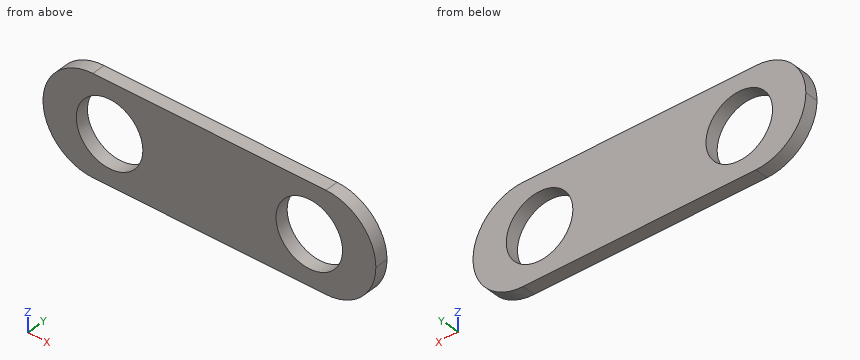
```python
from build123d import *

# Parameters (mm, degrees)
SKETCH1_W           = 50
SKETCH1_H           = 15
BOSS_EXTRUDE1_DEPTH = 2
SKETCH2_R           = 5
CUT_EXTRUDE1_DEPTH  = 2
CUT_EXTRUDE2_DEPTH  = 2


with BuildPart() as part:
    # Sketch1 → Boss-Extrude1 (new body)
    with BuildSketch(Plane(origin=(0, 0, 0), x_dir=(1, 0, 0), z_dir=(0, 1, 0))):
        with Locations((25, 7.5)):
            Rectangle(SKETCH1_W, SKETCH1_H)
    extrude(amount=BOSS_EXTRUDE1_DEPTH)

    # Sketch2 → Cut-Extrude1 (cut)
    with BuildSketch(Plane(origin=(0, 2, 0), x_dir=(1, 0, 0), z_dir=(0, 1, 0))):
        with Locations(Location((10, 7.5, 0), (0, 0, 270))):
            Circle(SKETCH2_R)
        with Locations(Location((40, 7.5, 0), (0, 0, 90))):
            Circle(SKETCH2_R)
    extrude(amount=-CUT_EXTRUDE1_DEPTH, mode=Mode.SUBTRACT)

    # Sketch5 → Cut-Extrude2 (cut)
    with BuildSketch(Plane(origin=(0, 2, 0), x_dir=(1, 0, 0), z_dir=(0, 1, 0))):
        with BuildLine():
            ThreePointArc((0, 7.5), (2.196699141, 12.803300859), (7.5, 15))
            Line((7.5, 15), (0, 15))
            Line((0, 15), (0, 7.5))
        make_face()
        with BuildLine():
            ThreePointArc((7.5, 0), (2.196699141, 2.196699141), (0, 7.5))
            Line((0, 7.5), (0, 0))
            Line((0, 0), (7.5, 0))
        make_face()
        with BuildLine():
            Line((50, 15), (42.5, 15))
            ThreePointArc((42.5, 15), (47.803300859, 12.803300859), (50, 7.5))
            Line((50, 7.5), (50, 15))
        make_face()
        with BuildLine():
            Line((50, 0), (50, 7.5))
            ThreePointArc((50, 7.5), (47.803300859, 2.196699141), (42.5, 0))
            Line((42.5, 0), (50, 0))
        make_face()
    extrude(amount=-CUT_EXTRUDE2_DEPTH, mode=Mode.SUBTRACT)


solid = part.part
```
Geometry: final body of the model. Coordinates: model frame, mm. Give positions to 0.01 mm unless a question says otherwise; leave off trailing zeros. Write each loop counter-clockwise with the first axis right and the second up, starting at its lowest first coordinate (ties: lowest second). Pieces come first, ordered by that corner, then holes.
1. Section query A-A, the plane x = 40. Return loops of the section in (y, z).
2. Section query D-D, the plane z = -9.25. Return loops of the section in (x, y).
3. Line query: probe 1 along X at (y, z) = (0.9, -7.5); probe 2 along X at (y, z) = (1.4, -11.5); probe 3 along Z at (x, y) = (40, 1.4). Output: solid intervals per line, ascending.
4. Section query C-C, the plane z = -5. Return loops of the section in (x, y), then the cut area to 3 significant figures.
5. Section query B-B, the plane y = 0.8. Return loops of the section in (x, z), then the cut area to 3 significant figures.
Computed:
1. outline: (0, -15) - (2, -15) - (2, -12.5) - (0, -12.5) - close; (0, -2.5) - (2, -2.5) - (2, 0) - (0, 0) - close
2. outline: (0.21, 0) - (5.32, 0) - (5.32, 2) - (0.21, 2) - close; (14.68, 0) - (35.32, 0) - (35.32, 2) - (14.68, 2) - close; (44.68, 0) - (49.79, 0) - (49.79, 2) - (44.68, 2) - close
3. probe 1: x = 0 to 5, 15 to 35, 45 to 50
3. probe 2: x = 1.16 to 7, 13 to 37, 43 to 48.84
3. probe 3: z = -15 to -12.5, -2.5 to 0
4. outline: (0.43, 0) - (5.67, 0) - (5.67, 2) - (0.43, 2) - close; (14.33, 0) - (35.67, 0) - (35.67, 2) - (14.33, 2) - close; (44.33, 0) - (49.57, 0) - (49.57, 2) - (44.33, 2) - close
4. area: 63.6 mm2
5. outline: (7.5, -15) - (42.5, -15) arc R7.5 ccw to (42.5, 0) - (7.5, 0) arc R7.5 ccw to start; hole circle Ø10 at (10, -7.5); hole circle Ø10 at (40, -7.5)
5. area: 545 mm2
